Answer from the drawing. Dimensions are ordinates in mm from the lowest x, y and z of the part. Give positions to 0.01 mm unless a question says otherwise; leave off trailing zeros. Write each loop counter-clockwise with the first axis right and the second up, starting at its lowest first coordinate (ties: lowest second). Pieces come first, ordered by that corner, then holes. Notation, with made-up numbers: (65, 64) -> (81, 64) arc R25 ccw to (81, 86) -> close; hole circle Ø2 at (43.25, -13). An arc over 180 degrees is marked (long way). Use a Markdown table: item, result. Add a question column.
Q1. Each of these flat-tipped pins is pushed along its axis until it touches: pin 1 Ø3 at (x, y) = (36.5, 36.5) entering from +Z; pin 2 Ø4.5 at (x, y) = (36.5, 5.5) entering from -Z. Where does it stop, or does it pass through?
Q2. Section C-C, the plane y = 21 is taken. Give the vertices of the cut face in (x, z), plus the area to 3 significant figures.
Q3. Consider line 1 (Y direction, x = 36.5, z = 5.25); line 2 (X direction, y = 37.5, z = 4.5). Determine where each line is inside the solid, lowest interval first.
Q4. Section D-D, the plane z = 4.5 is taken. Give the vertices of the cut face in (x, y), plus the area to 3 significant figures.
Q5. Section A-A, the plane y = 5.5 is taken. Give the vertices of the cut face in (x, z), plus the area to 3 significant figures.
Q6. For a pull along X with two mould halves and no side action, classify the marked faces 1, 2 and 3 as pulls with the +X half, pulls with the -X half, needs draft (parallel to the pull), parting line crosses it, or undercut.
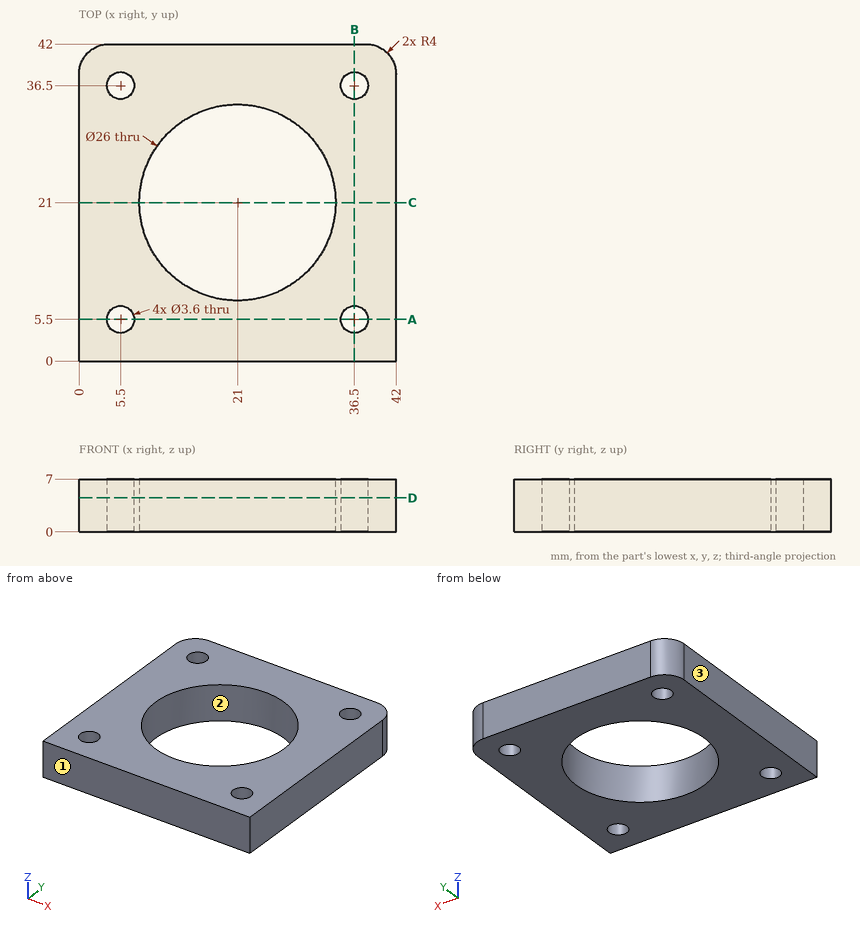
Result set:
| question | item | result |
|---|---|---|
| 1 | pin 1 | passes through |
| 1 | pin 2 | stops at z = 0 |
| 2 | outline | (0, 0) -> (8, 0) -> (8, 7) -> (0, 7) -> close; (34, 0) -> (42, 0) -> (42, 7) -> (34, 7) -> close |
| 2 | area | 112 mm2 |
| 3 | line 1 | y = 0 to 3.7, 7.3 to 34.7, 38.3 to 42 |
| 3 | line 2 | x = 0 to 4, 7 to 35, 38 to 42 |
| 4 | outline | (0, 0) -> (42, 0) -> (42, 38) arc R4 ccw to (38, 42) -> (4, 42) arc R4 ccw to (0, 38) -> close; hole circle Ø3.6 at (5.5, 5.5); hole circle Ø3.6 at (5.5, 36.5); hole circle Ø26 at (21, 21); hole circle Ø3.6 at (36.5, 5.5); hole circle Ø3.6 at (36.5, 36.5) |
| 4 | area | 1,190 mm2 |
| 5 | outline | (0, 0) -> (3.7, 0) -> (3.7, 7) -> (0, 7) -> close; (7.3, 0) -> (34.7, 0) -> (34.7, 7) -> (7.3, 7) -> close; (38.3, 0) -> (42, 0) -> (42, 7) -> (38.3, 7) -> close |
| 5 | area | 244 mm2 |
| 6 | face 1 | needs draft |
| 6 | face 2 | undercut |
| 6 | face 3 | pulls with the -X half |
